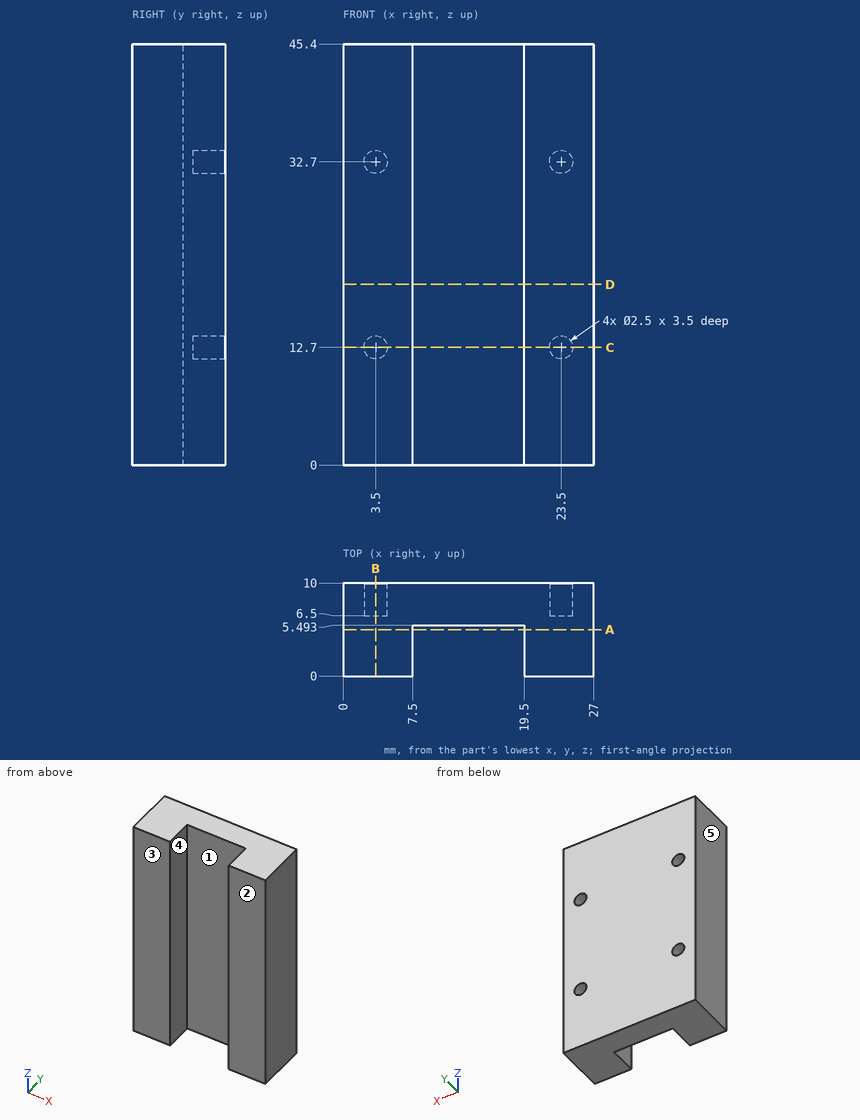
Input: dimensioned drawing with shaded views. Units: mm. Origin: part minimum x, y, z. A direction names the side the tool comes from. Give positions to 0.01 mm unless a question says otherwise; leave off trailing zeros. Write each loop counter-clockwise with the first axis right and the second up, starting at its lowest first coordinate (ties: lowest second). Pieces come first, ordered by that corner, then holes. Notation, with made-up numbers: (-9.75, 64) -> (40.25, 64) arc R24 ccw to (40.25, 94) -> close; hole circle Ø8 at (83, -17). An arc over 180 degrees is marked (long way). Answer as a JSON object with one key per item and string values.
1. Cut plane A-A on y = 5. Output: boundary loops of the cut face in (x, z).
Ans:
{"outline": "(0, 0) -> (7.5, 0) -> (7.5, 45.4) -> (0, 45.4) -> close; (19.5, 0) -> (27, 0) -> (27, 45.4) -> (19.5, 45.4) -> close"}
2. Cut plane D-D on z = 19.5. Output: boundary loops of the cut face in (x, y), and give its area (3 significant figures).
Ans:
{"outline": "(0, 0) -> (7.5, 0) -> (7.5, 5.49) -> (19.5, 5.49) -> (19.5, 0) -> (27, 0) -> (27, 10) -> (0, 10) -> close", "area": "204 mm^2"}
3. Contact query for flat-ended pins moving along their axis: pin 1 (2 mm diameter, centred on x = 3.5, z = 32.7, fed in from +Y); pin 2 (2 mm diameter, centred on x = 10.5, z = 25.5, fed in from -Y). Output: stop coordinate, or through.
Ans:
{"pin 1": "stops at y = 6.5", "pin 2": "stops at y = 5.49"}
4. Ray query, probe 1 along X at (y, z) = (9.2, 32.7); probe 2 along Z at (x, y) = (23.5, 8.5); probe 3 along X at (y, z) = (4, 42). Return the intervals inside material, ascending. Write a range as from..to.
Ans:
{"probe 1": "x = 0..2.25, 4.75..22.25, 24.75..27", "probe 2": "z = 0..11.45, 13.95..31.45, 33.95..45.4", "probe 3": "x = 0..7.5, 19.5..27"}
5. Mould query, pull axis X, two halves, no side actions, for the marked faces 3, 4 and 5. Classes: pulls with the +X half, pulls with the -X half, needs draft (parallel to the pull), parting line crosses it, or undercut.
Ans:
{"face 3": "needs draft", "face 4": "undercut", "face 5": "pulls with the -X half"}
6. Cut plane B-B on x = 3.5. Output: boundary loops of the cut face in (y, z).
Ans:
{"outline": "(0, 0) -> (10, 0) -> (10, 11.45) -> (6.5, 11.45) -> (6.5, 13.95) -> (10, 13.95) -> (10, 31.45) -> (6.5, 31.45) -> (6.5, 33.95) -> (10, 33.95) -> (10, 45.4) -> (0, 45.4) -> close"}
7. Cut plane C-C on z = 12.7. Output: boundary loops of the cut face in (x, y), and give its area (3 significant figures).
Ans:
{"outline": "(0, 0) -> (7.5, 0) -> (7.5, 5.49) -> (19.5, 5.49) -> (19.5, 0) -> (27, 0) -> (27, 10) -> (24.75, 10) -> (24.75, 6.5) -> (22.25, 6.5) -> (22.25, 10) -> (4.75, 10) -> (4.75, 6.5) -> (2.25, 6.5) -> (2.25, 10) -> (0, 10) -> close", "area": "187 mm^2"}
8. Access query for the marked faces 1 and 2. Directions: +Z, -Z, +X, -X, +Y, -Y. A direction counts if a zero-diameter tool reaches every point of the face in a straight line with its end or side. Return the directions, or none.
Ans:
{"face 1": "+Z, -Z, -Y", "face 2": "+Z, -Z, +X, -X, -Y"}
